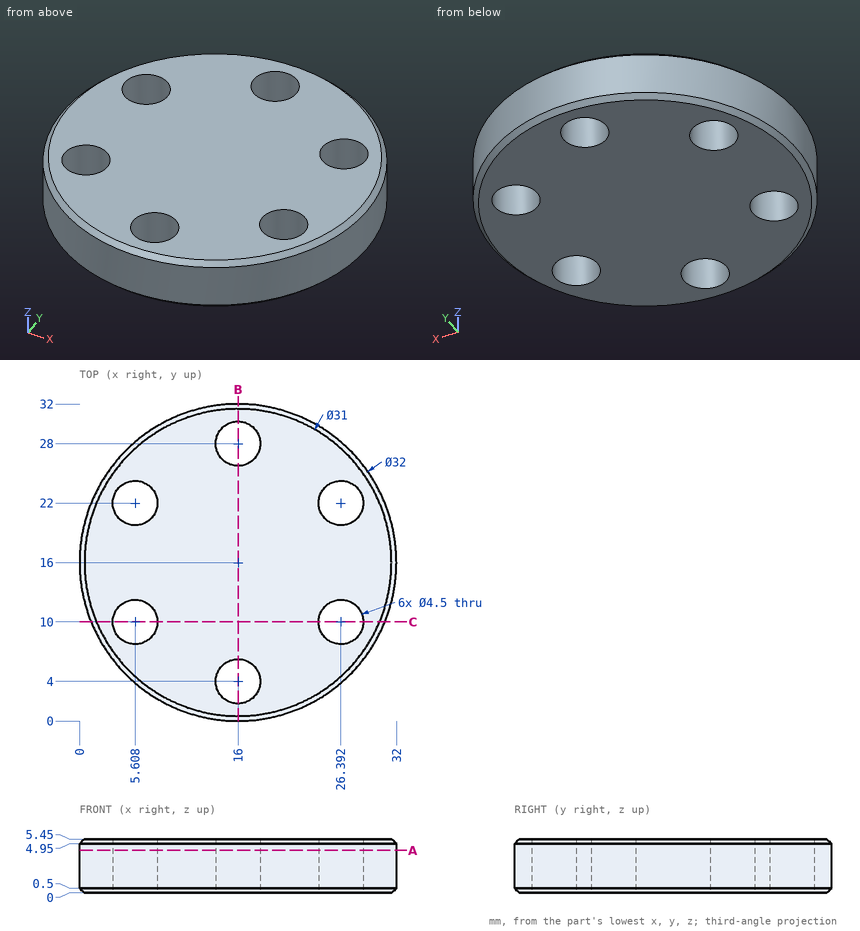
Answer from the drawing. Dimensions are ordinates in mm from the lowest x, y and z of the part. Coordinates: 2 decimals unless noted, no trailing zeros. Write each loop counter-clockwise with the first axis right and the second up, starting at its lowest first coordinate (ties: lowest second). Pieces come first, ordered by that corner, then holes. Notation, with made-up numbers: M -4,-39 L 26,-39 A13 ccw 26,-18 Z; hole C -18,57 d5. An arc over 180 degrees is marked long. Write item = value, one per line.
1. The part is cut by section A-A (z = 4.3). Determine the outline of the cut face in (x, y).
Solution:
outline = C 16,16 d32; hole C 5.61,10 d4.5; hole C 5.61,22 d4.5; hole C 16,4 d4.5; hole C 16,28 d4.5; hole C 26.39,10 d4.5; hole C 26.39,22 d4.5
2. Straight lines are drawn through the part: line 1 (Y direction, x = 16, z = 2.2); line 2 (X direction, y = 12, z = 4.8) (1 decimal); line 3 (X direction, y = 21.5, z = 0.75) (1 decimal). For each, find the intervals that lie inside material, in ascending order. Write a range as from..to.
Solution:
line_1 = 0..1.75, 6.25..25.75, 30.25..32
line_2 = 0.5..4.6, 6.6..25.4, 27.4..31.5
line_3 = 1..3.4, 7.8..24.2, 28.6..31
3. Flat-ended cylindrical pins translate along their axes: pin 1 (2.5 mm diameter, centred on x = 16, y = 4, fed in from -Z); pin 2 (1.5 mm diameter, centred on x = 18, z = 1.5, fed in from +Y); pin 3 (1.5 mm diameter, centred on y = 7, z = 5, fed in from +X); pin 4 (1 mm diameter, centred on y = 18.5, z = 3, fed in from +X). Find the tip coordinate at first contact, or state that the pin passes through.
Solution:
pin_1 = through
pin_2 = 31.95
pin_3 = 29.71
pin_4 = 31.87
4. The part is cut by section B-B (x = 16). Determine the outline of the cut face in (y, z).
Solution:
outline = M 0,0.5 L 0.5,0 L 1.75,0 L 1.75,5.45 L 0.5,5.45 L 0,4.95 Z; M 6.25,0 L 25.75,0 L 25.75,5.45 L 6.25,5.45 Z; M 30.25,0 L 31.5,0 L 32,0.5 L 32,4.95 L 31.5,5.45 L 30.25,5.45 Z
5. The part is cut by section C-C (y = 10). State how many separate pieces and enclosed holes the cut face has, then the cut area to 3 significant figures.
Solution:
separate_pieces = 3
enclosed_holes = 0
area = 112 mm2
